```python
from build123d import *

# Parameters (mm, degrees)
PAD002_DEPTH  = 8
SKETCH008_R   = 11
HOLE001_DEPTH = 8
SKETCH009_R   = 1.4
HOLE002_DEPTH = 8
SKETCH010_R   = 3.25
HOLE003_DEPTH = 1.7


with BuildPart() as part:
    # Sketch007 → Pad002 (new body)
    with BuildSketch(Plane.XY):
        with BuildLine():
            Line((-159, -1), (159, -1))
            ThreePointArc((162, -4), (161.12132, -1.87868), (159, -1))
            Line((162, -4), (162, -148))
            ThreePointArc((159, -151), (161.12132, -150.12132), (162, -148))
            Line((159, -151), (-159, -151))
            ThreePointArc((-162, -148), (-161.12132, -150.12132), (-159, -151))
            Line((-162, -148), (-162, -4))
            ThreePointArc((-159, -1), (-161.12132, -1.87868), (-162, -4))
        make_face()
    extrude(amount=PAD002_DEPTH)

    # Sketch008 → Hole001 (cut)
    with BuildSketch(Plane.XY):
        with Locations((-142.75, -17.7)):
            Circle(SKETCH008_R)
        with Locations((-120.25, -17.7)):
            Circle(SKETCH008_R)
        with Locations((-69.5, -37.5)):
            Circle(SKETCH008_R)
        with Locations((-69.5, -67.5)):
            Circle(SKETCH008_R)
        with Locations((-100, -77.5)):
            Circle(SKETCH008_R)
        with Locations((-125, -102.5)):
            Circle(SKETCH008_R)
        with Locations((-39.5, -77.5)):
            Circle(SKETCH008_R)
        with Locations((5, -80)):
            Circle(SKETCH008_R)
        with Locations((35, -70)):
            Circle(SKETCH008_R)
        with Locations((65, -65)):
            Circle(SKETCH008_R)
        with Locations((95, -70)):
            Circle(SKETCH008_R)
        with Locations((125, -75)):
            Circle(SKETCH008_R)
        with Locations((-10, -137.5)):
            Circle(SKETCH008_R)
        with Locations((20, -127.5)):
            Circle(SKETCH008_R)
        with Locations((35, -102.5)):
            Circle(SKETCH008_R)
        with Locations((65, -97.5)):
            Circle(SKETCH008_R)
        with Locations((95, -102.5)):
            Circle(SKETCH008_R)
        with Locations((125, -107.5)):
            Circle(SKETCH008_R)
    extrude(amount=HOLE001_DEPTH, mode=Mode.SUBTRACT)

    # Sketch009 → Hole002 (cut)
    with BuildSketch(Plane.XY):
        with Locations((0, -210)):
            Circle(SKETCH009_R)
        with Locations((160, -210)):
            Circle(SKETCH009_R)
        with Locations((160, -10)):
            Circle(SKETCH009_R)
        with Locations((-160, -210)):
            Circle(SKETCH009_R)
        with Locations((-160, -10)):
            Circle(SKETCH009_R)
        with Locations((0, -110)):
            Circle(SKETCH009_R)
    extrude(amount=HOLE002_DEPTH, mode=Mode.SUBTRACT)

    # Sketch010 → Hole003 (cut)
    with BuildSketch(Plane(origin=(0, 0, 8), x_dir=(-1, 0, 0), z_dir=(0, 0, 1))):
        with Locations((0, 110)):
            Circle(SKETCH010_R)
    extrude(amount=-HOLE003_DEPTH, mode=Mode.SUBTRACT)


with BuildPart() as part_1:
    # Body001 placement: moved
    add(part.part.moved(Location((0, 0, 6.71))))


solid = part_1.part
```
Verification items for the finished model (mm, model axes). A direction names the side the tool comes from. Round coordinates to 2 decimals unless told otherwise and drop trailing zeros. Order: outer loops, then holes, each group sorted by start corner. A loop starts at its lowest first (then second) coordinate and runs counter-clockwise, first axis right, second up.
1) Cross-section at C-C, the plane x = -142.75. Record the cut outline in (y, z), plus the area to 3 significant figures.
Geometry says:
outline: (-151, 6.71) - (-28.7, 6.71) - (-28.7, 14.71) - (-151, 14.71) - close; (-6.7, 6.71) - (-1, 6.71) - (-1, 14.71) - (-6.7, 14.71) - close
area: 1,020 mm2
2) Cross-section at B-B, the plane y = -37.5. Record the cut outline in (x, z), plus the area to 3 significant figures.
Geometry says:
outline: (-162, 6.71) - (-80.5, 6.71) - (-80.5, 14.71) - (-162, 14.71) - close; (-58.5, 6.71) - (162, 6.71) - (162, 14.71) - (-58.5, 14.71) - close
area: 2,420 mm2
3) Tool access check on faces 1 (the cylindrical face through (3.568, -69.094, 10.654)), 2 (the flat face through (-0.7, -108.6, 13.01)). Record the directions out of +Z, -Z, +X, -X, +Y, -Y that give a thin tool (end or side, any length) a straight path to the whole face; none if there is none.
Geometry says:
face 1: +Z, -Z
face 2: +Z
4) Draft check along X on faces 3 (the flat face through (2, -151, 11)), 4 (the cylindrical face through (-11.432, -126.594, 10.654)), 5 (the flat face through (-162, -77, 11)). Enter one of: +X half, -X half, draft (parallel to the pull), parting line (faces both ways), or undercut.
Geometry says:
face 3: draft
face 4: undercut
face 5: -X half
5) Cross-section at A-A, the plane x = 65. Record the cut outline in (y, z).
Geometry says:
outline: (-151, 6.71) - (-108.5, 6.71) - (-108.5, 14.71) - (-151, 14.71) - close; (-86.5, 6.71) - (-76, 6.71) - (-76, 14.71) - (-86.5, 14.71) - close; (-54, 6.71) - (-1, 6.71) - (-1, 14.71) - (-54, 14.71) - close
6) Depth check by flat-ended pin: pin 1 (17.5 mm diameter, centred on x = 20, y = -127.5, fed in from -Z); pin 2 (3 mm diameter, centred on x = 1.5, y = -109.5, fed in from +Z). Enter the tip coordinate at first touch or a pass-through.
Geometry says:
pin 1: passes through
pin 2: stops at z = 13.01
7) Material ranges on line 1 (Y direction, x = 126, z = 10.75); line 2 (Y direction, x = 129, z = 13.75); line 3 (X direction, y = -21, z = 7.5), recorded low to high.
Geometry says:
line 1: y = -151 to -118.45, -96.55 to -85.95, -64.05 to -1
line 2: y = -151 to -117.75, -97.25 to -85.25, -64.75 to -1
line 3: x = -162 to -153.24, -132.26 to -130.74, -109.76 to 162
8) Cross-section at D-D, the plane y = -17.7. Record the cut outline in (x, z), plus the area to 3 significant figures.
Geometry says:
outline: (-162, 6.71) - (-153.75, 6.71) - (-153.75, 14.71) - (-162, 14.71) - close; (-131.75, 6.71) - (-131.25, 6.71) - (-131.25, 14.71) - (-131.75, 14.71) - close; (-109.25, 6.71) - (162, 6.71) - (162, 14.71) - (-109.25, 14.71) - close
area: 2,240 mm2
